Check sheet for the modelled part. Datum: model origin and axes. Units: mm. Coordinates: 2 decimals unless noted, no trailing zeros. Loops run counter-clockwise (first coordinate to the right, second up) from the corner with the lowest first, then second, coordinate; pieces in that order, holes last. Notation, with made-up numbers: (-22.75, -17.75) - (13.25, -17.75) arc R18 ccw to (13.25, 5.25) - close; hole circle Ø10 at (60, 7.25). An arc over 180 degrees is marked (long way). Use a Markdown table: item, result. Add a question column.
1) Go/stop test with flat-tipped pins: P1, Ø1, axis at x = 46, z = 1.5, coming from the +Y side; P2, Ø3, axis at y = 45.5, z = 2.5, coming from the +X side; P3, Ø1, axis at x = 46, z = 4.5, coming from the -Y side. Record where each tip stops, or that it passes through.
2) Sectioned sample at C-C, the plane y = -38.5. Enter the section's corners in (x, z).
3) Sectioned sample at D-D, the plane x = 59. Enter the section's corners in (y, z), then the cut area to 3 significant figures.
4) Thickness scan on line 1 (Y direction, x = 76.2, z = 3); line 2 (X direction, y = -1.5, z = 0.75); line 3 (Y direction, x = 0, z = 4.25). Record the ranges inside material, lowest first.
5) Draft check along X on faces 1 (the cylindrical face through (0.756, 63.495, 3.131)), 2 (the flat face through (46, 1, 6.35)), 3 (the cylindrical face through (42.397, -13.352, 3.131)). Enter one of: pulls with the +X half, pulls with the -X half, needs draft (parallel to the pull), parting line crosses it, or undercut.
6) Sectioned sample at B-B, the plane x = -76.2. Enter the section's corners in (y, z).
7) Sectioned sample at A-A, the plane z = 4.75. Enter the section's corners in (x, y), then the cut area to 3 significant figures.
from build123d import *

# Parameters (mm, degrees)
F0_R     = 12.7
F1_DEPTH = 6.35


with BuildPart() as f1:
    # F0 (on Top) → F1 (new body)
    with BuildSketch(Plane.XY):
        with BuildLine():
            ThreePointArc((-63.5, 0), (-62.0954029096, 13.2819779212), (-57.94375, 25.976370723))
            ThreePointArc((-57.94375, 25.976370723), (-65.2892675199, 29.8164118691), (-73.3783848407, 31.6243733202))
            ThreePointArc((-73.3783848407, 31.6243733202), (-107.95, 0), (-73.3783848407, -31.6243733202))
            ThreePointArc((-73.3783848407, -31.6243733202), (-65.2892675199, -29.8164118691), (-57.94375, -25.976370723))
            ThreePointArc((-57.94375, -25.976370723), (-62.0954029096, -13.2819779212), (-63.5, 0))
        make_face()
        with Locations((-76.2, 0)):
            Circle(F0_R, mode=Mode.SUBTRACT)
        with BuildLine():
            ThreePointArc((-57.94375, -25.976370723), (-48.024670033, -14.636026826), (-44.45, 0))
            ThreePointArc((-44.45, 0), (-48.024670033, 14.636026826), (-57.94375, 25.976370723))
            ThreePointArc((-57.94375, 25.976370723), (-62.0954029096, 13.2819779212), (-63.5, 0))
            ThreePointArc((-63.5, 0), (-62.0954029096, -13.2819779212), (-57.94375, -25.976370723))
        make_face()
        with BuildLine():
            ThreePointArc((57.94375, -25.976370723), (48.024670033, -14.636026826), (44.45, 0))
            ThreePointArc((44.45, 0), (0, -44.45), (-44.45, 0))
            ThreePointArc((-44.45, 0), (-48.024670033, -14.636026826), (-57.94375, -25.976370723))
            ThreePointArc((-57.94375, -25.976370723), (-53.4352444367, -34.3063354497), (-47.7378395074, -41.8730065694))
            ThreePointArc((-47.7378395074, -41.8730065694), (0, -63.5), (47.7378395074, -41.8730065694))
            ThreePointArc((47.7378395074, -41.8730065694), (53.4352444367, -34.3063354497), (57.94375, -25.976370723))
        make_face()
        with BuildLine():
            ThreePointArc((-47.7378395074, -41.8730065694), (-53.4352444367, -34.3063354497), (-57.94375, -25.976370723))
            ThreePointArc((-57.94375, -25.976370723), (-65.2892675199, -29.8164118691), (-73.3783848407, -31.6243733202))
            ThreePointArc((-73.3783848407, -31.6243733202), (-59.5969903083, -34.344106995), (-47.7378395074, -41.8730065694))
        make_face()
        with BuildLine():
            ThreePointArc((-73.3783848407, 31.6243733202), (-65.2892675199, 29.8164118691), (-57.94375, 25.976370723))
            ThreePointArc((-57.94375, 25.976370723), (-53.4352444367, 34.3063354497), (-47.7378395074, 41.8730065694))
            ThreePointArc((-47.7378395074, 41.8730065694), (-59.5969903083, 34.344106995), (-73.3783848407, 31.6243733202))
        make_face()
        with BuildLine():
            ThreePointArc((-44.45, 0), (0, 44.45), (44.45, 0))
            ThreePointArc((44.45, 0), (48.024670033, 14.636026826), (57.94375, 25.976370723))
            ThreePointArc((57.94375, 25.976370723), (53.4352444367, 34.3063354497), (47.7378395074, 41.8730065694))
            ThreePointArc((47.7378395074, 41.8730065694), (0, 63.5), (-47.7378395074, 41.8730065694))
            ThreePointArc((-47.7378395074, 41.8730065694), (-53.4352444367, 34.3063354497), (-57.94375, 25.976370723))
            ThreePointArc((-57.94375, 25.976370723), (-48.024670033, 14.636026826), (-44.45, 0))
        make_face()
        with BuildLine():
            ThreePointArc((73.3783848407, 31.6243733202), (65.2892675199, 29.8164118691), (57.94375, 25.976370723))
            ThreePointArc((57.94375, 25.976370723), (62.0954029096, 13.2819779212), (63.5, 0))
            ThreePointArc((63.5, 0), (62.0954029096, -13.2819779212), (57.94375, -25.976370723))
            ThreePointArc((57.94375, -25.976370723), (65.2892675199, -29.8164118691), (73.3783848407, -31.6243733202))
            ThreePointArc((73.3783848407, -31.6243733202), (97.6298415614, -23.4270013159), (107.95, 0))
            ThreePointArc((107.95, 0), (97.6298415614, 23.4270013159), (73.3783848407, 31.6243733202))
        make_face()
        with BuildLine():
            ThreePointArc((88.9, 0), (76.2, -12.7), (63.5, 0))
            ThreePointArc((63.5, 0), (76.2, 12.7), (88.9, 0))
        make_face(mode=Mode.SUBTRACT)
        with BuildLine():
            ThreePointArc((57.94375, 25.976370723), (48.024670033, 14.636026826), (44.45, 0))
            ThreePointArc((44.45, 0), (48.024670033, -14.636026826), (57.94375, -25.976370723))
            ThreePointArc((57.94375, -25.976370723), (62.0954029096, -13.2819779212), (63.5, 0))
            ThreePointArc((63.5, 0), (62.0954029096, 13.2819779212), (57.94375, 25.976370723))
        make_face()
        with BuildLine():
            ThreePointArc((47.7378395074, 41.8730065694), (53.4352444367, 34.3063354497), (57.94375, 25.976370723))
            ThreePointArc((57.94375, 25.976370723), (65.2892675199, 29.8164118691), (73.3783848407, 31.6243733202))
            ThreePointArc((73.3783848407, 31.6243733202), (59.5969903083, 34.344106995), (47.7378395074, 41.8730065694))
        make_face()
        with BuildLine():
            ThreePointArc((73.3783848407, -31.6243733202), (65.2892675199, -29.8164118691), (57.94375, -25.976370723))
            ThreePointArc((57.94375, -25.976370723), (53.4352444367, -34.3063354497), (47.7378395074, -41.8730065694))
            ThreePointArc((47.7378395074, -41.8730065694), (59.5969903083, -34.344106995), (73.3783848407, -31.6243733202))
        make_face()
    extrude(amount=F1_DEPTH)


solid = f1.part
Solved:
| question | item | result |
|---|---|---|
| 1 | P1 | stops at y = 44.29 |
| 1 | P2 | stops at x = 45.78 |
| 1 | P3 | stops at y = -44.29 |
| 2 | outline | (-51.9, 0) - (-22.22, 0) - (-22.22, 6.35) - (-51.9, 6.35) - close; (22.22, 0) - (51.9, 0) - (51.9, 6.35) - (22.22, 6.35) - close |
| 3 | outline | (-34.59, 0) - (34.59, 0) - (34.59, 6.35) - (-34.59, 6.35) - close |
| 3 | area | 439 mm2 |
| 4 | line 1 | y = -31.75 to -12.7, 12.7 to 31.75 |
| 4 | line 2 | x = -107.91 to -88.81, -63.59 to -44.42, 44.42 to 63.59, 88.81 to 107.91 |
| 4 | line 3 | y = -63.5 to -44.45, 44.45 to 63.5 |
| 5 | face 1 | parting line crosses it |
| 5 | face 2 | needs draft |
| 5 | face 3 | undercut |
| 6 | outline | (-31.75, 0) - (-12.7, 0) - (-12.7, 6.35) - (-31.75, 6.35) - close; (12.7, 0) - (31.75, 0) - (31.75, 6.35) - (12.7, 6.35) - close |
| 7 | outline | (-73.38, -31.62) arc R38.1 cw to (-47.74, -41.87) arc R63.5 ccw to (47.74, -41.87) arc R38.1 cw to (73.38, -31.62) arc R31.75 ccw (long way) to (73.38, 31.62) arc R38.1 cw to (47.74, 41.87) arc R63.5 ccw to (-47.74, 41.87) arc R38.1 cw to (-73.38, 31.62) arc R31.75 ccw (long way) to start; hole circle Ø25.4 at (-76.2, 0); hole circle Ø88.9 at (0, 0); hole circle Ø25.4 at (76.2, 0) |
| 7 | area | 10,700 mm2 |
